from build123d import *

# Parameters (mm, degrees)
F0_R          = 104.775
F1_DEPTH      = 114.3
F1_DEPTH_BACK = 114.3
F2_R          = 76.2
F3_DEPTH      = 19.05
F4_R          = 22.225


with BuildPart() as f1:
    # F0 (on Right) → F1 (new body, two sides)
    with BuildSketch(Plane.YZ) as f1_sk:
        Circle(F0_R)
    extrude(amount=F1_DEPTH)
    extrude(f1_sk.sketch, amount=-F1_DEPTH_BACK)

    # F2 (on face) → F3 (join)
    with BuildSketch(Plane(origin=(-114.3, 0, 0), x_dir=(0, -1, 0), z_dir=(-1, 0, 0))):
        Circle(F2_R)
    extrude(amount=F3_DEPTH)

    # F4
    f4_edges = [f1.edges().sort_by_distance(p)[0] for p in [
        (-114.3, -104.775, 0),
        (114.3, -104.775, 0),
    ]]
    fillet(f4_edges, radius=F4_R)


solid = f1.part
Work out the finished part from the listing and answer in its coordinate system (mm). A direction names the side the tool comes from. Give positions to 0.01 mm unless a question says otherwise; leave off trailing zeros. Loops run counter-clockwise (first coordinate to the right, second up) from the corner with the lowest first, then second, coordinate; pieces in that order, holes last. Notation, with made-up numbers: (49.25, 37.25) -> (59.25, 37.25) arc R22 cw to (59.25, 63.25) -> close; hole circle Ø4 at (81, 77.5). An arc over 180 degrees is marked (long way). Use a Markdown table: item, result. Add a question column.
1. For faces 1 (the cylindrical face through (-123.692, 60.47, -46.367)), 2 (the flat face through (-133.35, 1, 1)), determine the directions among +Z, -Z, +X, -X, +Y, -Y from which every point of the face is accessible in a straight line to the end or side of a thin tool.
2. Find the intervals of material crossed by probe 1 along X at (y, z) = (43.5, -66); probe 2 along X at (y, z) = (-92, 36.5); probe 3 along Y at (x, z) = (30, 93.5), in increasing order.
3. Flat-ended cylindrical pins translate along their axes: pin 1 Ø10 at (x, y) = (-49.5, -13) entering from +Z; pin 2 Ø1 at (x, z) = (-103, -2) entering from -Y; pin 3 Ø12 at (x, z) = (-81, -27.5) entering from -Y. Find the tip coordinate at first contact, or state that the pin passes through.
4. Section A-A on z = 0 is taken. Determine the outline of the cut face in (x, y) (3 decimals).
5. Section C-C on x = 41 is taken. Determine the outline of the cut face in (y, z) (3 decimals).
Results below:
| question | item | result |
|---|---|---|
| 1 | face 1 | -X |
| 1 | face 2 | +Z, -Z, -X, +Y, -Y |
| 2 | probe 1 | x = -114.3 to 114.3 |
| 2 | probe 2 | x = -107.05 to 107.05 |
| 2 | probe 3 | y = -47.28 to 47.28 |
| 3 | pin 1 | stops at z = 104.47 |
| 3 | pin 2 | stops at y = -102.16 |
| 3 | pin 3 | stops at y = -102.55 |
| 4 | outline | (-133.35, -76.2) -> (-114.3, -76.2) -> (-114.3, -82.55) arc R22.225 ccw to (-92.075, -104.775) -> (92.075, -104.775) arc R22.225 ccw to (114.3, -82.55) -> (114.3, 82.55) arc R22.225 ccw to (92.075, 104.775) -> (-92.075, 104.775) arc R22.225 ccw to (-114.3, 82.55) -> (-114.3, 76.2) -> (-133.35, 76.2) -> close |
| 5 | outline | circle Ø209.55 at (0, 0) |
